The listing builds one solid part. Answer for the finished solid, in the listing's coordinates (mm). A direction names the side the tool comes from. Coordinates: 2 decimals unless noted, no trailing zeros. Order: outer loops, then holes, each group sorted by start corner. A loop starts at its lowest first (then second) coordinate and runs counter-clockwise, first axis right, second up. Notation, with made-up numbers: M -38.5,-36.75 L 0.5,-36.75 A6 cw 0.5,-32.75 Z; hole C 22,5.5 d7. An arc over 180 degrees is marked long. One line per item, written item: value. Start each with the question number.
Q1. For faces 1 (the flat face through (25.4, -13, 3)), 2 (the flat face through (6, -13, 0)), determine the directions among +Z, -Z, +X, -X, +Y, -Y from which every point of the face is accessible in a straight line to the end or side of a thin tool.
Q2. Straight lines are drawn through the part: line 1 along Z through (x, y) = (21, -14.75); line 2 along X through (y, z) = (-10, 2); line 3 along X through (y, z) = (-9, 3). For each, find the intervals that lie inside material, in ascending order. Write a range as [from, to].
Q3. The part is cut by section B-B on x = 17.5. Give the vertices of the cut face in (y, z), then the cut area to 3 significant figures.
Q4. Each of these flat-tipped pins is pushed along its axis until it touches: pin 1 Ø10 at (y, z) = (-18, 16) entering from +X; pin 2 Ø6.5 at (x, y) = (21.5, -12.5) entering from -Z; pin 3 Ø5 at (y, z) = (-9.5, 4) entering from +X. Where does it stop, or does it pass through?
Q5. The part is cut by section C-C on z = 22.5. Give the vertices of the cut face in (x, y).
Q6. The part is cut by section A-A on y = -21. Give the vertices of the cut face in (x, z).
Q7. Determine the mould class of faces 3 (the flat face through (19, 0, 16)), 4 (the flat face through (19, -13, 6.35)), 5 (the flat face through (6.298, -12.878, 15.653)) for opening direction X: pulls with the +X half, pulls with the -X half, needs draft (parallel to the pull), parting line crosses it, or undercut.
```python
from build123d import *

# Parameters (mm, degrees)
F0_W      = 38.1
F0_H      = 31.75
F2_DEPTH  = 25.4
F7_W      = 12.7
F7_H      = 6.35
F8_DEPTH  = 25.4
F10_DEPTH = 25.4
F12_DEPTH = 25.4


# Not quite as in the source:
# - the program builds the solid bodies; features that only make, move or delete a surface that nothing else refers to are left out


with BuildPart() as f2:
    # F0 (on Front) → F2 (new body)
    with BuildSketch(Plane.XZ):
        with Locations((19.05, 15.875)):
            Rectangle(F0_W, F0_H)
    extrude(amount=F2_DEPTH)

    # F7 (on face) → F8 (cut)
    with BuildSketch(Plane.XZ.offset(25.4)):
        with Locations((19.05, 3.175)):
            Rectangle(F7_W, F7_H)
    extrude(amount=-F8_DEPTH, mode=Mode.SUBTRACT)

    # F9 (on face) → F10 (cut)
    with BuildSketch(Plane.XZ.offset(25.4)):
        Polygon((0, 31.75), (0, 0), (12.7748493105, 31.75), align=None)
    extrude(amount=-F10_DEPTH, mode=Mode.SUBTRACT)

    # F11 (on face) → F12 (cut)
    with BuildSketch(Plane.XZ.offset(25.4)):
        Polygon((25.4374246553, 31.75), (38.1, 0), (38.1, 31.75), align=None)
    extrude(amount=-F12_DEPTH, mode=Mode.SUBTRACT)


solid = f2.part
```
Output:
1. face 1: -Z, +Y, -Y
1. face 2: -Z, +X, -X, +Y, -Y
2. line 1: z = [6.35, 31.75]
2. line 2: x = [0.8, 12.7], [25.4, 37.3]
2. line 3: x = [1.21, 12.7], [25.4, 36.9]
3. outline: M -25.4,6.35 L 0,6.35 L 0,31.75 L -25.4,31.75 Z
3. area: 645 mm^2
4. pin 1: stops at x = 33.71
4. pin 2: stops at z = 6.35
4. pin 3: stops at x = 37.5
5. outline: M 9.05,-25.4 L 29.13,-25.4 L 29.13,0 L 9.05,0 Z
6. outline: M 0,0 L 12.7,0 L 12.7,6.35 L 25.4,6.35 L 25.4,0 L 38.1,0 L 25.44,31.75 L 12.77,31.75 Z
7. face 3: needs draft
7. face 4: undercut
7. face 5: pulls with the -X half
